from build123d import *

# Parameters (mm, degrees)
SKETCH1_R           = 4
SKETCH1_R_2         = 1.6
BOSS_EXTRUDE1_DEPTH = 4
SKETCH2_W           = 26
SKETCH2_H           = 4
BOSS_EXTRUDE2_DEPTH = 33
SKETCH3_R           = 5
SKETCH3_R_2         = 1.6
CUT_EXTRUDE1_DEPTH  = 33
CUT_EXTRUDE2_DEPTH  = 33
CUT_EXTRUDE3_DEPTH  = 5
SKETCH7_W           = 26
SKETCH7_H           = 15.618281376
CUT_EXTRUDE4_DEPTH  = 5
FILLET1_R           = 5
CUT_EXTRUDE5_DEPTH  = 10


with BuildPart() as part:
    # Sketch1 → Boss-Extrude1 (new body)
    with BuildSketch(Plane.XY):
        with BuildLine():
            Line((13, -10), (-13, -10))
            Line((-13, -10), (-13, 10))
            ThreePointArc((-13, 10), (0, 23), (13, 10))
            Line((13, 10), (13, -10))
        make_face()
        with Locations((0, 10)):
            Circle(SKETCH1_R, mode=Mode.SUBTRACT)
        with Locations((-8.5, 10)):
            Circle(SKETCH1_R_2, mode=Mode.SUBTRACT)
        with Locations(Location((8.5, 10, 0), (0, 0, 180))):
            Circle(SKETCH1_R_2, mode=Mode.SUBTRACT)
    extrude(amount=BOSS_EXTRUDE1_DEPTH)

    # Sketch2 → Boss-Extrude2 (add)
    with BuildSketch(Plane.XY.offset(4)):
        with Locations((0, -8)):
            Rectangle(SKETCH2_W, SKETCH2_H)
    extrude(amount=BOSS_EXTRUDE2_DEPTH)

    # Sketch3 → Cut-Extrude1 (cut)
    with BuildSketch(Plane.XZ.offset(10)):
        with Locations((0, 21)):
            Circle(SKETCH3_R)
        with Locations((-8, 25.5)):
            Circle(SKETCH3_R_2)
        with Locations(Location((8, 25.5, 0), (0, 0, 270))):
            Circle(SKETCH3_R_2)
        with Locations((8, 11.5)):
            Circle(SKETCH3_R_2)
        with Locations(Location((-8, 11.5, 0), (0, 0, 270))):
            Circle(SKETCH3_R_2)
    extrude(amount=-CUT_EXTRUDE1_DEPTH, mode=Mode.SUBTRACT)

    # Sketch4 → Cut-Extrude2 (cut)
    with BuildSketch(Plane.XY.offset(4)):
        with BuildLine():
            Line((-10.1, 5), (-10.1, 15))
            ThreePointArc((-10.1, 15), (-8.5, 16.6), (-6.9, 15))
            Line((-6.9, 15), (-6.9, 5))
            ThreePointArc((-6.9, 5), (-8.5, 3.4), (-10.1, 5))
        make_face()
        with BuildLine():
            Line((10.1, 5), (10.1, 15))
            ThreePointArc((10.1, 15), (8.5, 16.6), (6.9, 15))
            Line((6.9, 15), (6.9, 5))
            ThreePointArc((6.9, 5), (8.5, 3.4), (10.1, 5))
        make_face()
    extrude(amount=-CUT_EXTRUDE2_DEPTH, mode=Mode.SUBTRACT)

    # Sketch6 → Cut-Extrude3 (cut)
    with BuildSketch(Plane(origin=(0, -6, 0), x_dir=(1, 0, 0), z_dir=(0, 1, 0))):
        with BuildLine():
            Line((6.42648755, -15.03229904), (6.42648755, -7.96770096))
            ThreePointArc((6.42648755, -7.96770096), (8, -6.39418851), (9.57351245, -7.96770096))
            Line((9.57351245, -7.96770096), (9.57351245, -15.03229904))
            ThreePointArc((9.57351245, -15.03229904), (8, -16.60581149), (6.42648755, -15.03229904))
        make_face()
        with BuildLine():
            Line((-6.42648755, -15.03229904), (-6.42648755, -7.96770096))
            ThreePointArc((-6.42648755, -7.96770096), (-8, -6.39418851), (-9.57351245, -7.96770096))
            Line((-9.57351245, -7.96770096), (-9.57351245, -15.03229904))
            ThreePointArc((-9.57351245, -15.03229904), (-8, -16.60581149), (-6.42648755, -15.03229904))
        make_face()
    extrude(amount=-CUT_EXTRUDE3_DEPTH, mode=Mode.SUBTRACT)

    # Sketch7 → Cut-Extrude4 (cut)
    with BuildSketch(Plane(origin=(0, -6, 0), x_dir=(1, 0, 0), z_dir=(0, 1, 0))):
        with Locations((0, -29.190859312)):
            Rectangle(SKETCH7_W, SKETCH7_H)
    extrude(amount=-CUT_EXTRUDE4_DEPTH, mode=Mode.SUBTRACT)

    # Fillet1
    # the kernel refuses this fillet: 5 mm, written as the material it takes off along each edge
    with BuildSketch(Plane(origin=(-13, 6.5, 21.381718624), x_dir=(0, 0, -1), z_dir=(0, -1, 0))) as fillet1_piece_1:
        with BuildLine():
            CenterArc((FILLET1_R, FILLET1_R), FILLET1_R, 180, 90)
            Line((0, FILLET1_R), (0, 0))
            Line((0, 0), (FILLET1_R, 0))
        make_face()
    extrude(amount=29, mode=Mode.SUBTRACT)
    with BuildSketch(Plane(origin=(13, 6.5, 21.381718624), x_dir=(0, 0, -1), z_dir=(0, -1, 0))) as fillet1_piece_2:
        with BuildLine():
            CenterArc((FILLET1_R, -FILLET1_R), FILLET1_R, 90, 90)
            Line((0, -FILLET1_R), (0, 0))
            Line((0, 0), (FILLET1_R, 0))
        make_face()
    extrude(amount=29, mode=Mode.SUBTRACT)
    with BuildSketch(Plane(origin=(4.985407796, 3.710716282, 21.381718624), x_dir=(-0.20045131167218372, 0, -0.9797036652217348), z_dir=(0, -1, 0))) as fillet1_piece_3:
        with BuildLine():
            CenterArc((4.119908, 4.807706292), FILLET1_R, 191.563351745, 62.494863063)
            Line((-0.778610326, 3.805449733), (0, 0))
            ThreePointArc((0, 0), (1.373302667, 0.192293708), (2.746605333, 0))
        make_face()
    extrude(amount=23.421432563, mode=Mode.SUBTRACT)
    with BuildSketch(Plane(origin=(-4.985407796, 3.710716282, 21.381718624), x_dir=(-1, 0, 0), z_dir=(0, -1, 0))) as fillet1_piece_4:
        with BuildLine():
            CenterArc((3.884286513, 5), FILLET1_R, 207.505136937, 62.494863063)
            ThreePointArc((-0.550560642, 2.690859312), (-0.08688947, 1.383975182), (0, 0))
            Line((0, 0), (3.884286513, 0))
        make_face()
    extrude(amount=23.421432563, mode=Mode.SUBTRACT)

    # Sketch8 → Cut-Extrude5 (cut)
    with BuildSketch(Plane(origin=(0, 0, 0), x_dir=(-1, 0, 0), z_dir=(0, 0, -1))):
        with BuildLine():
            Line((-4, 5), (-4, 15))
            ThreePointArc((-4, 15), (0, 19), (4, 15))
            Line((4, 15), (4, 5))
            ThreePointArc((4, 5), (0, 1), (-4, 5))
        make_face()
    extrude(amount=-CUT_EXTRUDE5_DEPTH, mode=Mode.SUBTRACT)


solid = part.part
Build history of the part. All positions in model axes, mm. A direction names the side the tool comes from. Coordinates: 2 decimals unless noted, no trailing zeros. Order: outer loops, then holes, each group sorted by start corner. A loop starts at its lowest first (then second) coordinate and runs counter-clockwise, first axis right, second up. Notation, with made-up numbers: (54, 69) -> (94, 69) arc R5 ccw to (94, 77) -> close; hole circle Ø3 at (55, 64). An arc over 180 degrees is marked (long way). One line per item, written item: value.
(1) Drop flat-ended pins along their axis: pin 1 Ø5 at (x, y) = (-10, -1.5) entering from +Z; pin 2 Ø2 at (y, z) = (18.5, 3) entering from -X; pin 3 Ø1.5 at (y, z) = (-3.5, 7) entering from -X; pin 4 Ø6 at (x, z) = (-7.5, 4) entering from +Y. Give the stop position or say it passes through.
Checked values:
pin 1: z = 4
pin 2: x = -10.62
pin 3: through
pin 4: y = 22.2
(2) Mould opens along X. For faces 1 (the flat face through (-9.574, -8, 10)), 2 (the flat face through (0, -1, 0)), 3 (the cylindrical face through (0, 23, 2)) say: pulls with the +X half, pulls with the -X half, needs draft (parallel to the pull), parting line crosses it, or undercut.
Checked values:
face 1: undercut
face 2: needs draft
face 3: parting line crosses it
(3) Probe line 1 (X direction, y = 7.5, z = 3); line 2 (X direction, y = 15, z = 1.75); line 3 (Z direction, x = 0.5, y = -4). List the from-to ranges inside material, lowest first. Write a range as [from, to].
Checked values:
line 1: [-13, -10.1], [-6.9, -4], [4, 6.9], [10.1, 13]
line 2: [-12, -10.1], [-6.9, -4], [4, 6.9], [10.1, 12]
line 3: [0, 4]
(4) Tool access for faces 4 (the flat face through (9.574, -8, 10)), 5 (the cylindrical face through (-11.65, -7.97, 19.8)), 6 (the flat face through (4, 10, 2)): list every direction of +Z, -Z, +X, -X, +Y, -Y with a clear straight run to the whole face (end or side of a thin tool).
Checked values:
face 4: +Y, -Y
face 5: +Z, -X, +Y, -Y
face 6: +Z, -Z
(5) Slice it at B-B, the plane z = 8.75. List the corners of the cut face in (x, y).
Checked values:
outline: (-13, -10) -> (-9.57, -10) -> (-9.57, -6) -> (-13, -6) -> close; (-6.43, -10) -> (6.43, -10) -> (6.43, -6) -> (-6.43, -6) -> close; (9.57, -10) -> (13, -10) -> (13, -6) -> (9.57, -6) -> close
(6) Slice it at D-D, the plane z = 2. List the corners of the cut face in (x, y), plus the area to 3 significant figures.
Checked values:
outline: (-13, -10) -> (13, -10) -> (13, 10) arc R13 ccw to (-13, 10) -> close; hole (-10.1, 5) arc R1.6 ccw to (-6.9, 5) -> (-6.9, 15) arc R1.6 ccw to (-10.1, 15) -> close; hole (-4, 5) arc R4 ccw to (4, 5) -> (4, 15) arc R4 ccw to (-4, 15) -> close; hole (6.9, 5) arc R1.6 ccw to (10.1, 5) -> (10.1, 15) arc R1.6 ccw to (6.9, 15) -> close
area: 575 mm2
(7) Slice it at A-A, the plane y = 8. List the corners of the cut face in (x, z).
Checked values:
outline: (-13, 0) -> (-10.1, 0) -> (-10.1, 4) -> (-13, 4) -> close; (-6.9, 0) -> (-4, 0) -> (-4, 4) -> (-6.9, 4) -> close; (4, 0) -> (6.9, 0) -> (6.9, 4) -> (4, 4) -> close; (10.1, 0) -> (13, 0) -> (13, 4) -> (10.1, 4) -> close
(8) Slice it at C-C, the plane x = -1. List the corners of the cut face in (y, z).
Checked values:
outline: (-10, 0) -> (1.13, 0) -> (1.13, 4) -> (-6, 4) -> (-6, 16.1) -> (-10, 16.1) -> close; (18.87, 0) -> (22.96, 0) -> (22.96, 4) -> (18.87, 4) -> close
